Design review of the part built by this model. Coordinates are the model's own, in mm. A direction names the side the tool comes from. Give positions to 0.01 mm unless a question says otherwise; leave off trailing zeros. Write each loop counter-clockwise with the first axis right and the second up, starting at its lowest first coordinate (ties: lowest second). Pieces come first, ordered by that corner, then holes. Notation, with made-up numbers: (-31.5, -1.75) -> (-5.5, -1.75) arc R25 cw to (-5.5, 13.25) -> close; hole circle Ø5 at (69, 58.25). An arc over 180 degrees is marked (long way). Put each result on its own line as item: value. Start each with the question number.
Autodesk Inventor part; units mm, degrees
ref_plane "YZ Plane" through (0, 0, 0) normal (1, 0, 0) x (0, 1, 0)
ref_plane "XZ Plane" through (0, 0, 0) normal (0, 1, 0) x (-1, 0, 0)
ref_plane "XY Plane" through (0, 0, 0) normal (0, 0, 1) x (1, 0, 0)
sketch "Skizze1" plane through (0, 0, 0) normal (0, 0, 1) x (1, 0, 0)
  line L0 (52.5, 37.5) -> (-52.5, 37.5)
  line L1 (-52.5, 37.5) -> (-52.5, -37.5)
  line L2 (-52.5, -37.5) -> (52.5, -37.5)
  line L3 (52.5, -37.5) -> (52.5, 37.5)
  line L4 (52.5, 37.5) -> (-52.5, -37.5) construction
  line L5 (-52.5, 37.5) -> (52.5, -37.5) construction
  point P0 (0, 0)
  dimension "d0" = 105
  dimension "d1" = 75
extrude "Extrusion1" add sketch "Skizze1" along normal blind 2.5
fillet "Rundung1" radius 2 4 edges at (-52.5, 37.5, 1.25) (52.5, 37.5, 1.25) (52.5, -37.5, 1.25) (-52.5, -37.5, 1.25)
sketch "Skizze2" plane through (0, 0, 2.5) normal (0, 0, 1) x (1, 0, 0)
  arc A0 (-52.5, -35.5) -> (-50.5, -37.5) centre (-50.5, -35.5) ccw construction
  line L0 (-50.5, -37.5) -> (50.5, -37.5) construction
  arc A1 (50.5, -37.5) -> (52.5, -35.5) centre (50.5, -35.5) ccw construction
  line L1 (52.5, -35.5) -> (52.5, 35.5) construction
  arc A2 (52.5, 35.5) -> (50.5, 37.5) centre (50.5, 35.5) ccw construction
  line L2 (50.5, 37.5) -> (-50.5, 37.5) construction
  arc A3 (-50.5, 37.5) -> (-52.5, 35.5) centre (-50.5, 35.5) ccw construction
  line L3 (-52.5, 35.5) -> (-52.5, -35.5) construction
  line L4 (-50, 35) -> (50, 35) construction
  line L5 (50, 35) -> (50, -35) construction
  line L6 (50, -35) -> (-50, -35) construction
  line L7 (-50, -35) -> (-50, 35) construction
  line L8 (-50, 35) -> (50, -35) construction
  line L9 (50, 35) -> (-50, -35) construction
  line L10 (-50, 35) -> (-47.5, 35) construction
  line L11 (-50, 35) -> (-50, 32.5) construction
  line L12 (50, 35) -> (47.5, 35) construction
  line L13 (50, 35) -> (50, 32.5) construction
  line L14 (-50, -35) -> (-50, -32.5) construction
  line L15 (-47.5, 35) -> (-47.5, -3) construction
  line L16 (-50, 32.5) -> (-30, 32.5) construction
  line L17 (50, 32.5) -> (32, 32.5) construction
  line L18 (50, -35) -> (47.5, -35) construction
  line L19 (47.5, -35) -> (47.5, -32.5) construction
  circle A4 centre (-30, 32.5) radius 4
  circle A5 centre (32, 32.5) radius 4
  circle A6 centre (47.5, -32.5) radius 4
  circle A7 centre (-47.5, -3) radius 4
  circle A8 centre (-30, 32.5) radius 1.15
  circle A9 centre (32, 32.5) radius 1.15
  circle A10 centre (47.5, -32.5) radius 1.15
  circle A11 centre (-47.5, -3) radius 1.15
  point P0 (0, 0)
  dimension "d5" = 100
  dimension "d6" = 70
  dimension "d7" = 2.5
  dimension "d8" = 2.5
  dimension "d9" = 2.5
  dimension "d10" = 2.5
  dimension "d11" = 2.5
  dimension "d12" = 38
  dimension "d13" = 20
  dimension "d14" = 18
  dimension "d15" = 2.5
  dimension "d16" = 2.5
  dimension "d17" = 8
  dimension "d18" = 8
  dimension "d19" = 8
  dimension "d20" = 8
  dimension "d23" = 2.3
  dimension "d24" = 2.3
  dimension "d25" = 2.3
  dimension "d26" = 2.3
extrude "Extrusion3" add sketch "Skizze2" along normal blind 15
sketch "Skizze3" plane through (0, 0, 2.5) normal (0, 0, 1) x (1, 0, 0)
  circle A0 centre (47.5, -32.5) radius 4 construction
  circle A1 centre (-30, 32.5) radius 4 construction
  circle A2 centre (32, 32.5) radius 4 construction
  circle A3 centre (-47.5, -3) radius 4 construction
  arc A4 (-52.5, -35.5) -> (-50.5, -37.5) centre (-50.5, -35.5) ccw construction
  line L0 (-50.5, -37.5) -> (50.5, -37.5) construction
  arc A5 (50.5, -37.5) -> (52.5, -35.5) centre (50.5, -35.5) ccw construction
  line L1 (52.5, -35.5) -> (52.5, 35.5) construction
  arc A6 (52.5, 35.5) -> (50.5, 37.5) centre (50.5, 35.5) ccw construction
  line L2 (50.5, 37.5) -> (-50.5, 37.5) construction
  arc A7 (-50.5, 37.5) -> (-52.5, 35.5) centre (-50.5, 35.5) ccw construction
  line L3 (-52.5, 35.5) -> (-52.5, -35.5) construction
  line L4 (-47.5, 25) -> (47.5, 25) construction
  line L5 (47.5, 25) -> (47.5, -25) construction
  line L6 (47.5, -25) -> (-47.5, -25) construction
  line L7 (-47.5, -25) -> (-47.5, 25) construction
  line L8 (-47.5, 25) -> (47.5, -25) construction
  line L9 (47.5, 25) -> (-47.5, -25) construction
  point P0 (0, 0)
  dimension "d29" = 50
hole "Bohrung1" at (-47.5, 25, 2.5) at (47.5, 25, 2.5) at (47.5, -25, 2.5) at (-47.5, -25, 2.5) direction (0, 0, -1) diameter 4.2 end through all
properties part number "PCB_Case_Btm"
Q1. Machinability: for faces 1 (the face through (-30, 33, 2.5)), 2 (the face through (49.363, 24.031, 1.232)), which of the approach directions +Z, -Z, +X, -X, +Y, -Y give a long, thin tool a straight path to every point of the face, cutting with its end or side? Answer none if there is none.
Q2. Take a section at C-C on x = -47.5. Give the boundary of the cut face in (y, z), then the cut area to 3 significant figures.
Q3. Take a section at B-B on y = -25. Give the boundary of the cut face in (x, z), then the cut area to 4 significant figures.
Q4. Mouldability with a two-part tool opening along Y and no side actions: class faces 3 (the face through (-45.637, 24.031, 1.232)), 4 (the face through (-51.9, 36.93, 1.27)), 5 (the face through (51.9, -36.93, 1.27)) as +Y half, -Y half, draft (parallel to the pull), parting line (faces both ways), or undercut.
Q5. To check wall thickness, follow probe 1 along X at (y, z) = (-25, 1.8); probe 2 along Y at (x, z) = (47.5, 1.55); probe 3 along Y at (x, z) = (32, 6). State the ranges of each line that lie inside material, in increasing order. Write a range as from..to.
Q6. For pin 1 (2 mm diameter, centred on x = -30, y = 32.5, fed in from +Z); pin 2 (1 mm diameter, centred on y = 2.5, z = 4.5, fed in from -X), all flat-tipped, find the tip position at first contact; note any pin that passes through.
Q7. Take a section at D-D on y = -3. Give the boundary of the cut face in (x, z).
Q8. Take a section at A-A on z = 9.5. Give the boundary of the cut face in (x, y), then the cut area to 3 significant figures.
Result:
1. face 1: +Z
1. face 2: +Z, -Z
2. outline: (-37.5, 0) -> (-27.1, 0) -> (-27.1, 2.5) -> (-37.5, 2.5) -> close; (-22.9, 0) -> (22.9, 0) -> (22.9, 2.5) -> (1, 2.5) -> (1, 17.5) -> (-1.85, 17.5) -> (-1.85, 2.5) -> (-4.15, 2.5) -> (-4.15, 17.5) -> (-7, 17.5) -> (-7, 2.5) -> (-22.9, 2.5) -> close; (27.1, 0) -> (37.5, 0) -> (37.5, 2.5) -> (27.1, 2.5) -> close
2. area: 252 mm^2
3. outline: (-52.5, 0) -> (-49.6, 0) -> (-49.6, 2.5) -> (-52.5, 2.5) -> close; (-45.4, 0) -> (45.4, 0) -> (45.4, 2.5) -> (-45.4, 2.5) -> close; (49.6, 0) -> (52.5, 0) -> (52.5, 2.5) -> (49.6, 2.5) -> close
3. area: 241.5 mm^2
4. face 3: undercut
4. face 4: +Y half
4. face 5: -Y half
5. probe 1: x = -52.5..-49.6, -45.4..45.4, 49.6..52.5
5. probe 2: y = -37.5..-27.1, -22.9..22.9, 27.1..37.5
5. probe 3: y = 28.5..31.35, 33.65..36.5
6. pin 1: stops at z = 2.5
6. pin 2: passes through
7. outline: (-52.5, 0) -> (52.5, 0) -> (52.5, 2.5) -> (-43.5, 2.5) -> (-43.5, 17.5) -> (-46.35, 17.5) -> (-46.35, 2.5) -> (-48.65, 2.5) -> (-48.65, 17.5) -> (-51.5, 17.5) -> (-51.5, 2.5) -> (-52.5, 2.5) -> close
8. outline: circle Ø8 at (-47.5, -3); circle Ø8 at (-30, 32.5); circle Ø8 at (32, 32.5); circle Ø8 at (47.5, -32.5); hole circle Ø2.3 at (-47.5, -3); hole circle Ø2.3 at (-30, 32.5); hole circle Ø2.3 at (32, 32.5); hole circle Ø2.3 at (47.5, -32.5)
8. area: 184 mm^2
